The listing builds one solid part. Answer for the finished solid, in the listing's coordinates (mm). A direction names the side the tool comes from. Give positions to 0.01 mm unless a question says otherwise; leave off trailing zeros. Order: outer loops, then holes, each group sorted by start corner. A loop starts at its lowest first (then second) coordinate and runs counter-clockwise, first axis right, second up. Notation, with made-up numbers: (-7.5, -29.75) - (29.5, -29.75) arc R14 ccw to (29.5, -10.75) - close; hole circle Ø3 at (-19.5, -4.5). An arc over 180 degrees is marked (long way). Use a Markdown table: item, result. Add a question column.
1) Flat-ended cylindrical pins translate along their axes: pin 1 (1 mm diameter, centred on x = 46, y = -25.5, fed in from +Z); pin 2 (3 mm diameter, centred on x = -74, y = -22, fed in from +Z); pin 3 (0.6 mm diameter, centred on y = 31.5, z = 26.5, fed in from -X). Find the tip coordinate at first contact, or state that the pin passes through.
2) Find section B-B, the plane z = 3. Determine the outline of the cut face in (x, y).
3) For faces 4 (the face through (73.7, 10.9, 22.5)), 5 (the face through (-74, -18.5, 24)), 6 (the face through (-74, -6.9, 9)), 7 (the face through (-1, 36, 14)), determine the directions among +Z, -Z, +X, -X, +Y, -Y from which every point of the face is accessible in a straight line to the end or side of a thin tool.
4) The mould has two halves that part along X. Classify faces 1 (the face through (71.7, 1, 14)), 2 (the face through (-74.8, -39.14, 10.79)), 3 (the face through (-74, 6.5, 9)): released by +X, released by -X, zero draft, split by the parting line, or undercut.
5) Find section A-A, the plane x = 25.82. Determine the outline of the cut face in (y, z), plus the area to 3 significant figures.
6) Find section C-C, the plane x = -4.66. Determine the outline of the cut face in (y, z).
7) Straight lines are drawn through the part: line 1 (Y direction, x = -4.66, z = -0.45); line 2 (X direction, y = -24.13, z = -0.7); line 3 (X direction, y = 31.5, z = 3). For each, find the intervals that lie inside material, in ascending order.
8) Find section D-D, the plane x = -28.5. Determine the outline of the cut face in (y, z).
Solid Edge part; units mm, degrees
sketch "Sketch1" plane through (0, 0, 0) normal (0, 0, 1) x (1, 0, 0)
  line L0 (-75.7, -40) -> (75.7, -40)
  line L1 (75.7, -40) -> (75.7, 40)
  line L2 (75.7, 40) -> (-75.7, 40)
  line L3 (-75.7, 40) -> (-75.7, -40)
  dimension "D1" = 75.7
extrude "Protrusion1" add sketch "Sketch1" against normal blind 4
sketch "Sketch2" plane through (0, 0, 0) normal (0, 0, 1) x (1, 0, 0)
  line L0 (-75.7, 40) -> (75.7, 40)
  line L1 (75.7, 40) -> (75.7, -40)
  line L2 (75.7, -40) -> (-75.7, -40)
  line L3 (-75.7, -40) -> (-75.7, 40)
  line L4 (-71.7, 36) -> (71.7, 36)
  line L5 (71.7, 36) -> (71.7, -36)
  line L6 (71.7, -36) -> (-71.7, -36)
  line L7 (-71.7, -36) -> (-71.7, 36)
extrude "ExtrudedProtrusion_2" add sketch "Sketch2" along normal blind 26
sketch "Sketch3" plane through (-71.7, 0, 8) normal (1, 0, 0) x (0, 1, 0)
  line L0 (-6.9, -3.5) -> (6.5, -3.5)
  line L1 (6.5, -3.5) -> (6.5, 5.5)
  line L2 (6.5, 5.5) -> (-6.9, 5.5)
  line L3 (-6.9, 5.5) -> (-6.9, -3.5)
  dimension "D1" = 6.9
  dimension "D2" = 6.9
extrude "Cutout1" cut sketch "Sketch3" against normal up to next
sketch "Sketch4" plane through (-75.7, 0, 11) normal (-1, 0, 0) x (0, -1, 0)
  line L0 (7.5, 15) -> (-3, 15)
  line L1 (-3, 15) -> (-3, 9)
  line L2 (-3, 9) -> (7.5, 9)
  line L3 (7.5, 9) -> (7.5, 15)
  line L4 (29, 15) -> (18.5, 15)
  line L5 (18.5, 15) -> (18.5, 9)
  line L6 (18.5, 9) -> (29, 9)
  line L7 (29, 9) -> (29, 15)
  line L8 (-12.5, 15) -> (-29, 15)
  line L9 (-29, 15) -> (-29, 12.5)
  line L10 (-29, 12.5) -> (-12.5, 12.5)
  line L11 (-12.5, 12.5) -> (-12.5, 15)
  dimension "D1" = 3
  dimension "D2" = 29
  dimension "D3" = 18.5
  dimension "D4" = 12.5
  dimension "D5" = 7.5
extrude "Cutout2" cut sketch "Sketch4" against normal up to next
sketch "Sketch5" plane through (71.7, 0, 13) normal (-1, 0, 0) x (0, -1, 0)
  circle A0 centre (-10.8, 13) radius 3.5
  dimension "D1" = 10.8
extrude "Cutout3" cut sketch "Sketch5" against normal up to next
sketch "Sketch6" plane through (0, 24.15, 26) normal (0, 0, 1) x (0, -1, 0)
  line L0 (16.85, 71.7) -> (60.15, 71.7)
  line L1 (60.15, 71.7) -> (60.15, -71.7)
  line L2 (60.15, -71.7) -> (53.15, -71.7)
  line L3 (53.15, -71.7) -> (53.15, -73.7)
  line L4 (62.15, -73.7) -> (53.15, -73.7)
  line L5 (62.15, 73.7) -> (62.15, -73.7)
  line L6 (16.85, 73.7) -> (62.15, 73.7)
  line L7 (16.85, 71.7) -> (16.85, 73.7)
  line L8 (-11.85, -71.7) -> (-11.85, 71.7)
  line L9 (-11.85, 71.7) -> (9.85, 71.7)
  line L10 (9.85, 73.7) -> (9.85, 71.7)
  line L11 (-13.85, 73.7) -> (9.85, 73.7)
  line L12 (-13.85, -73.7) -> (-13.85, 73.7)
  line L13 (-4.85, -73.7) -> (-13.85, -73.7)
  line L14 (-4.85, -73.7) -> (-4.85, -71.7)
  line L15 (-4.85, -71.7) -> (-11.85, -71.7)
  line L16 (21.15, -71.7) -> (11.65, -71.7)
  line L17 (11.65, -71.7) -> (11.65, -73.7)
  line L18 (21.15, -73.7) -> (11.65, -73.7)
  line L19 (21.15, -73.7) -> (21.15, -71.7)
  line L20 (31.65, -71.7) -> (31.65, -73.7)
  line L21 (42.65, -73.7) -> (31.65, -73.7)
  line L22 (42.65, -73.7) -> (42.65, -71.7)
  line L23 (42.65, -71.7) -> (31.65, -71.7)
extrude "Protrusion2" add sketch "Sketch6" along normal blind 2
hole "Hole_8" at (-55.46, 24.13, 0) direction (0, 0, -1) diameter 3 end up to next
hole "Hole1" at (-56.73, -24.13, 0) direction (0, 0, -1) diameter 3 end up to next
hole "Hole2" at (-4.66, 8.89, 0) direction (0, 0, -1) diameter 3 end up to next
hole "Hole3" at (-4.66, -19.05, 0) direction (0, 0, -1) diameter 3 end up to next
hole "Hole4" at (19.47, 24.13, 0) direction (0, 0, -1) diameter 3 end up to next
hole "Hole5" at (57.57, 14.61, 0) direction (0, 0, -1) diameter 3 end up to next
hole "Hole6" at (25.82, -24.13, 0) direction (0, 0, -1) diameter 3 end up to next
fillet "Round1" radius 3 4 edges at (-75.7, 40, 11) (-75.7, -40, 11) (75.7, -40, 11) (75.7, 40, 11)
chamfer "Chamfer1" distance 3 angle 45 7 edges at (24.32, -24.13, -4) (56.07, 14.61, -4) (17.97, 24.13, -4) (-6.16, 8.89, -4) (-6.16, -19.05, -4) (-56.96, 24.13, -4) (-58.23, -24.13, -4)
The answers:
| question | item | result |
|---|---|---|
| 1 | pin 1 | z = 0 |
| 1 | pin 2 | z = 20 |
| 1 | pin 3 | x = -73.7 |
| 2 | outline | (-75.7, -37) arc R3 ccw to (-72.7, -40) - (72.7, -40) arc R3 ccw to (75.7, -37) - (75.7, 37) arc R3 ccw to (72.7, 40) - (-72.7, 40) arc R3 ccw to (-75.7, 37) - close; hole (-71.7, -36) - (71.7, -36) - (71.7, 36) - (-71.7, 36) - close |
| 3 | face 4 | +Z, +X |
| 3 | face 5 | +Z, -X |
| 3 | face 6 | -X |
| 3 | face 7 | +Z |
| 4 | face 1 | undercut |
| 4 | face 2 | released by -X |
| 4 | face 3 | zero draft |
| 5 | outline | (-40, -4) - (-28.63, -4) - (-25.63, -1) - (-25.63, 0) - (-36, 0) - (-36, 28) - (-38, 28) - (-38, 26) - (-40, 26) - close; (-22.63, -1) - (-19.63, -4) - (40, -4) - (40, 26) - (38, 26) - (38, 28) - (36, 28) - (36, 0) - (-22.63, 0) - close |
| 5 | area | 515 mm2 |
| 6 | outline | (-40, -4) - (-23.55, -4) - (-20.55, -1) - (-20.55, 0) - (-36, 0) - (-36, 28) - (-38, 28) - (-38, 26) - (-40, 26) - close; (-17.55, -1) - (-14.55, -4) - (4.39, -4) - (7.39, -1) - (7.39, 0) - (-17.55, 0) - close; (10.39, -1) - (13.39, -4) - (40, -4) - (40, 26) - (38, 26) - (38, 28) - (36, 28) - (36, 0) - (10.39, 0) - close |
| 7 | line 1 | -40 to -20.55, -17.55 to 7.39, 10.39 to 40 |
| 7 | line 2 | -75.7 to -58.23, -55.23 to 24.32, 27.32 to 75.7 |
| 7 | line 3 | -75.7 to -71.7, 71.7 to 75.7 |
| 8 | outline | (-40, -4) - (40, -4) - (40, 26) - (38, 26) - (38, 28) - (36, 28) - (36, 0) - (-36, 0) - (-36, 28) - (-38, 28) - (-38, 26) - (-40, 26) - close |
